Check sheet for the modelled part. Datum: model origin and axes. Units: mm. A direction names the side the tool comes from. Round coordinates to 2 decimals unless told otherwise and drop trailing zeros. Order: outer loops, then holes, each group sorted by start corner. A loop starts at its lowest first (then second) coordinate and runs counter-clockwise, first axis right, second up.
```python
from build123d import *

# Parameters (mm, degrees)
SKETCH1_W            = 16.48
SKETCH1_H            = 27.0711
SKETCH1_W_2          = 12.48
SKETCH1_H_2          = 23.0711
BOSS_EXTRUDE1_DEPTH  = 17.2796
BOSS_EXTRUDE2_DEPTH  = 17.2796
SKETCH3_W            = 4.8956
SKETCH3_H            = 3.65
CUT_EXTRUDE1_DEPTH   = 27.853165612
SKETCH4_W            = 4
SKETCH4_H            = 5.15
BOSS_EXTRUDE3_DEPTH  = 17.2796
FILLET1_R            = 3
SKETCH5_W            = 1
SKETCH5_H            = 7.15
CUT_EXTRUDE3_DEPTH   = 31.685099533
M2_CLEARANCE_HOLE1_D = 2.4


with BuildPart() as part:
    # Sketch1 → Boss-Extrude1 (new body)
    with BuildSketch(Plane(origin=(0, 0, 0), x_dir=(0, 0, -1), z_dir=(1, 0, 0))):
        with Locations((0, -5.29555)):
            Rectangle(SKETCH1_W, SKETCH1_H)
        with Locations((0, -5.29555)):
            Rectangle(SKETCH1_W_2, SKETCH1_H_2, mode=Mode.SUBTRACT)
    extrude(amount=BOSS_EXTRUDE1_DEPTH)

    # Sketch2 → Boss-Extrude2 (add)
    with BuildSketch(Plane(origin=(17.2796, 0, 0), x_dir=(0, 0, -1), z_dir=(1, 0, 0))):
        Polygon((-5, 8.24), (5, 8.24), (3.5, 10.24), (-3.5, 10.24), align=None)
    extrude(amount=-BOSS_EXTRUDE2_DEPTH)

    # Sketch3 → Cut-Extrude1 (cut, through all)
    with BuildSketch(Plane(origin=(17.2796, 0, 0), x_dir=(0, 0, -1), z_dir=(1, 0, 0))):
        with Locations((0, 6.915)):
            Rectangle(SKETCH3_W, SKETCH3_H)
    extrude(amount=-CUT_EXTRUDE1_DEPTH, mode=Mode.SUBTRACT)

    # Sketch4 → Boss-Extrude3 (add)
    with BuildSketch(Plane(origin=(17.2796, 0, 0), x_dir=(0, 0, -1), z_dir=(1, 0, 0))):
        with Locations((0, -21.4061)):
            Rectangle(SKETCH4_W, SKETCH4_H)
    extrude(amount=-BOSS_EXTRUDE3_DEPTH)

    # Fillet1
    fillet1_edges = [part.edges().sort_by_distance(p)[0] for p in [
        (17.2796, -23.9811, 0),
        (0, -23.9811, 0),
    ]]
    fillet(fillet1_edges, radius=FILLET1_R)

    # Sketch5 → Cut-Extrude3 (cut, through all)
    with BuildSketch(Plane(origin=(17.2796, 0, 0), x_dir=(0, 0, -1), z_dir=(1, 0, 0))):
        with Locations((0, -20.4061)):
            Rectangle(SKETCH5_W, SKETCH5_H)
    extrude(amount=-CUT_EXTRUDE3_DEPTH, mode=Mode.SUBTRACT)

    # M2 Clearance Hole1 (through all)
    with Locations(Plane(origin=(0, 0, -2), x_dir=(-1, 0, 0), z_dir=(0, 0, -1))):
        with Locations((-14.2796, -20.9811), (-3, -20.9811)):
            Hole(M2_CLEARANCE_HOLE1_D / 2)


solid = part.part
```
Item 1: Go/stop test with flat-tipped pins: P1, Ø1.6, axis at x = 7.5, z = -7, coming from the +Y side; P2, Ø3, axis at x = 3, y = -20.98, coming from the +Z side; P3, Ø7, axis at x = 10.5, z = 6, coming from the -Y side. Record where each tip stops, or that it passes through.
Answer:
P1: stops at y = 8.24
P2: stops at z = 2
P3: stops at y = -18.83
Item 2: Sectioned sample at C-C (y = -12.5). Record the cut outline in (x, z), and give its area (3 significant figures).
Answer:
outline: (0, -8.24) - (17.28, -8.24) - (17.28, -6.24) - (0, -6.24) - close; (0, 6.24) - (17.28, 6.24) - (17.28, 8.24) - (0, 8.24) - close
area: 69.1 mm2
Item 3: Sectioned sample at A-A (y = 7.5). Record the cut outline in (x, z).
Answer:
outline: (0, -8.24) - (17.28, -8.24) - (17.28, -2.45) - (0, -2.45) - close; (0, 2.45) - (17.28, 2.45) - (17.28, 8.24) - (0, 8.24) - close
Item 4: Release check for a two-part mould opening along Z. For faces 1 (the flat face through (9, -20, 0.5)), 2 (the flat face through (9, -5, -8.24)), 3 (the cylindrical face through (0.855, -23.079, 1.24)), 4 (the flat face through (9, 7, -2.448)) record: released by +Z, released by -Z, zero draft, split by the parting line, or undercut.
Answer:
face 1: undercut
face 2: released by -Z
face 3: zero draft
face 4: undercut
Item 5: Access from +Z, -Z, +X, -X, +Y, -Y to the whole of each face (thin tool, end or side, straight path). Record for faces 5 (the flat face through (9, 8.24, -7)), 6 (the flat face through (9, -16.831, -3)), 7 (the flat face through (9, -20, -0.5)), 8 (the flat face through (9, -21, -2)), 9 (the flat face through (9, -18.831, 5)).
Answer:
face 5: -Z, +X, -X, +Y
face 6: +X, -X
face 7: +X, -X, -Y
face 8: -Z, +X, -X, -Y
face 9: +Z, +X, -X, -Y
Item 6: Sectioned sample at B-B (z = 1). Record the cut outline in (x, y), and give its area (3 significant figures).
Answer:
outline: (0, -20.98) arc R3 ccw to (3, -23.98) - (14.28, -23.98) arc R3 ccw to (17.28, -20.98) - (17.28, -16.83) - (0, -16.83) - close; (0, 8.74) - (17.28, 8.74) - (17.28, 10.24) - (0, 10.24) - close; hole circle Ø2.4 at (3, -20.98); hole circle Ø2.4 at (14.28, -20.98)
area: 137 mm2
Item 7: Scan lines: line 1 along Y through (x, z) = (3, -1.6); line 2 along Z through (x, y) = (15.5, -15.5); line 3 along Z through (x, y) = (7.5, 6.5). Record each from-to range of solid material in increasing order.
Answer:
line 1: y = -23.98 to -22.18, -19.78 to -16.83, 8.74 to 10.24
line 2: z = -8.24 to -6.24, 6.24 to 8.24
line 3: z = -8.24 to -2.45, 2.45 to 8.24
Item 8: Sectioned sample at D-D (x = 8.5). Record the cut outline in (y, z).
Answer:
outline: (-23.98, -2) - (-18.83, -2) - (-18.83, -8.24) - (8.24, -8.24) - (8.24, -5) - (10.24, -3.5) - (10.24, 3.5) - (8.24, 5) - (8.24, 8.24) - (-18.83, 8.24) - (-18.83, 2) - (-23.98, 2) - (-23.98, 0.5) - (-16.83, 0.5) - (-16.83, 6.24) - (6.24, 6.24) - (6.24, 2.45) - (8.74, 2.45) - (8.74, -2.45) - (6.24, -2.45) - (6.24, -6.24) - (-16.83, -6.24) - (-16.83, -0.5) - (-23.98, -0.5) - close
